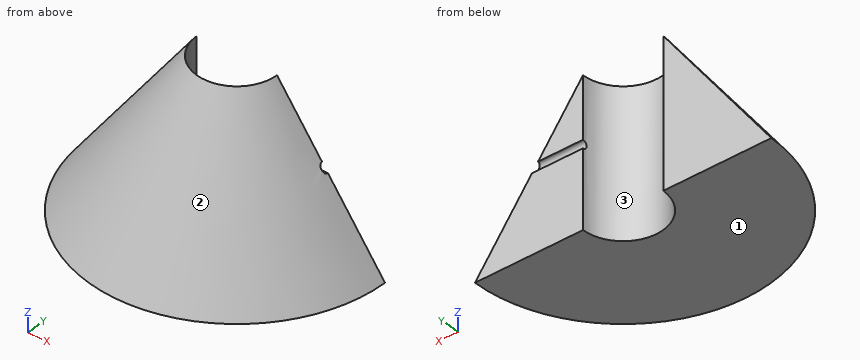
```python
from build123d import *

# Parameters (mm, degrees)
ENL_V_MAT_EXTRU_1_REACH = 313.769
ESQUISSE7_R             = 5


with BuildPart() as part:
    # Esquisse4 → Révolution1 (revolve)
    with BuildSketch(Plane(origin=(0, 0, 0), x_dir=(0, 0, -1), z_dir=(1, 0, 0)), mode=Mode.PRIVATE) as r_volution1_sk:
        Polygon((-180, 48.75), (0, 180), (0, 48.75), align=None)
    revolve(r_volution1_sk.sketch.rotate(Axis((0, 0, 180), (0, 0, -1)), 90), axis=Axis((0, 0, 180), (0, 0, -1)))

    # Enlèv. mat.-Extru.1: up to this cone (the profile starts inside it)
    enl_v_mat_extru_1_end = Plane(origin=(0, 0, 100), z_dir=(0, 0, -1)).offset(-146.857141857) * Cone(1e-06, 414.319409722, 568.20947519, align=(Align.CENTER, Align.CENTER, Align.MIN), mode=Mode.PRIVATE)
    # Esquisse7 → Enlèv. mat.-Extru.1 (cut, up to the surface)
    with BuildSketch(Plane(origin=(0, 0, 0), x_dir=(0, 0, -1), z_dir=(1, 0, 0)), mode=Mode.PRIVATE) as enl_v_mat_extru_1_sk1:
        with Locations(Location((-100, 0, 0), (0, 0, 180))):
            Circle(ESQUISSE7_R)
    enl_v_mat_extru_1_tool1 = extrude(enl_v_mat_extru_1_sk1.sketch, amount=ENL_V_MAT_EXTRU_1_REACH, mode=Mode.PRIVATE) & enl_v_mat_extru_1_end
    add(enl_v_mat_extru_1_tool1.solids().sort_by_distance((0, 0, 100))[0], mode=Mode.SUBTRACT)

    # Enlèv. mat.-Surface1
    split(bisect_by=Plane(origin=(0, 0, 0), x_dir=(1, 0, 0), z_dir=(0, 1, 0)), keep=Keep.BOTTOM)


solid = part.part
```
Could you check a few things on this model? Use its own coordinates, in mm. Face numbers are marked on the shaded views. Coordinates: 2 decimals unless noted, no trailing zeros. Order: outer loops, then holes, each group sorted by start corner. A loop starts at its lowest first (then second) coordinate and runs counter-clockwise, first axis right, second up. Notation, with made-up numbers: M -24.5,30 L 27.5,30 A12 cw 27.5,43 Z; hole C 41,73 d7. An arc over 180 degrees is marked long. Use a Markdown table: item, result. Add a question column.
Q1. I'm going to push flat-ended pins straight in: pin 1 (12 mm diameter, centred on x = -82.5, z = 55.5, fed in from -Y); pin 2 (8 mm diameter, centred on x = 19.5, y = -117, fed in from -Z); pin 3 (1.5 mm diameter, centred on x = 65.5, z = 117, fed in from -Y); pin 4 (5 mm diameter, centred on x = -38.5, z = 38.5, fed in from -Y). Where does each tip first touch, or does it pass through?
Q2. I want a section at B-B on z = 49.5. List the corners of the cut face in (x, y) for me, then the cut area to 3 significant figures.
Q3. We'd pull the mould along X, two halves only. Please class the marked faces 1, 2 and 3: pulls with the +X half, pulls with the -X half, needs draft (parallel to the pull), parting line crosses it, or undercut.
Q4. I want a section at C-C on z = 100. List the corners of the cut face in (x, y) for me, then the cut area to 3 significant figures.
Q5. If I drill on L1, parallel to Z at x = -38.5, y = -30; L2, parallel to Y at x = 4, z = 133.5; L3, parallel to X at y = -59, z = 117, over which ranges is the centre line in solid material (lowest first)?
Q6. I want a section at A-A on x = 0. List the corners of the cut face in (y, z) for me, then the cut area to 3 significant figures.
Checked values:
| question | item | result |
|---|---|---|
| 1 | pin 1 | y = -119.3 |
| 1 | pin 2 | z = 0 |
| 1 | pin 3 | y = -69.41 |
| 1 | pin 4 | y = -148.96 |
| 2 | outline | M -143.91,0 A143.91 ccw 143.91,0 L 48.75,0 A48.75 cw -48.75,0 Z |
| 2 | area | 28,800 mm² |
| 3 | face 1 | needs draft |
| 3 | face 2 | parting line crosses it |
| 3 | face 3 | undercut |
| 4 | outline | M -107.08,0 A107.08 ccw 106.97,-5 L 48.49,-5 A48.75 cw -48.75,0 Z |
| 4 | area | 14,000 mm² |
| 5 | L1 | 0 to 179.92 |
| 5 | L2 | -82.56 to -48.59 |
| 5 | L3 | -74.06 to 74.06 |
| 6 | outline | M -180,0 L -48.75,0 L -48.75,180 Z |
| 6 | area | 11,800 mm² |
